```python
from build123d import *

# Parameters (mm, degrees)
SKETCH1_W                    = 60
SKETCH1_H                    = 170
BASE_FLANGE1_DEPTH           = 4
EDGE_FLANGE1_STRIP_W         = 26
EDGE_FLANGE1_STRIP_H         = 4
EDGE_FLANGE1_STRIP_CUT_DEPTH = 170
EDGE_FLANGE1_DEPTH           = 170
SKETCH15_R                   = 10
CUT_EXTRUDE4_DEPTH           = 10
CUT_EXTRUDE5_DEPTH           = 10
FILLET1_R                    = 10
F_1_0MM_DOWEL_HOLE2_D        = 5.2
F_1_0MM_DOWEL_HOLE2_DEPTH    = 12.03
F_1_0MM_DOWEL_HOLE2_TIP      = 1.562237609
SKETCH33_R                   = 2.6
CUT_EXTRUDE6_DEPTH           = 7
F_1_0MM_DOWEL_HOLE3_D        = 5.2
F_1_0MM_DOWEL_HOLE3_DEPTH    = 12.03
F_1_0MM_DOWEL_HOLE3_TIP      = 1.562237609
CUT_EXTRUDE7_DEPTH           = 10


# Sheet-metal steps are written as plain solids
with BuildPart() as part:
    # Sketch1 → Base-Flange1 (new body)
    with BuildSketch(Plane(origin=(0, 0, 0), x_dir=(1, 0, 0), z_dir=(0, 1, 0))):
        Rectangle(SKETCH1_W, SKETCH1_H)
    extrude(amount=-BASE_FLANGE1_DEPTH)

    # Edge-Flange1 strip (across the edge) → Edge-Flange1 strip cut (cut)
    with BuildSketch(Plane(origin=(-30, 0, -85), x_dir=(1, 0, 0), z_dir=(0, 0, 1))):
        with Locations((-8, -2)):
            Rectangle(EDGE_FLANGE1_STRIP_W, EDGE_FLANGE1_STRIP_H)
    extrude(amount=EDGE_FLANGE1_STRIP_CUT_DEPTH, mode=Mode.SUBTRACT)

    # Edge-Flange1 section (across the edge) → Edge-Flange1 (add)
    with BuildSketch(Plane(origin=(-30, 0, -85), x_dir=(1, 0, 0), z_dir=(0, 0, 1))):
        with BuildLine():
            Line((-4, 5), (-4, 186))
            Line((-4, 186), (0, 186))
            Line((0, 186), (0, 5))
            ThreePointArc((0, 5), (1.464466094, 1.464466094), (5, 0))
            Line((5, 0), (5, -4))
            ThreePointArc((5, -4), (-1.363961031, -1.363961031), (-4, 5))
        make_face()
    extrude(amount=EDGE_FLANGE1_DEPTH)

    # Sketch15 → Cut-Extrude4 (cut)
    with BuildSketch(Plane(origin=(-30, 0, 0), x_dir=(0, 0, -1), z_dir=(1, 0, 0))):
        with Locations(Location((-43, 63, 0), (0, 0, 90))):
            Circle(SKETCH15_R)
        with Locations(Location((57, 143, 0), (0, 0, 90))):
            Circle(SKETCH15_R)
    extrude(amount=-CUT_EXTRUDE4_DEPTH, mode=Mode.SUBTRACT)

    # Sketch16 → Cut-Extrude5 (cut)
    with BuildSketch(Plane(origin=(-30, 0, 0), x_dir=(0, 0, -1), z_dir=(1, 0, 0))):
        Polygon((-85, 96), (45, 186), (-85, 186), align=None)
    extrude(amount=-CUT_EXTRUDE5_DEPTH, mode=Mode.SUBTRACT)

    # Fillet1
    fillet1_edges = [part.edges().sort_by_distance(p)[0] for p in [
        (-32, 186, -85),
        (-32, 186, -45),
        (-32, 96, 85),
        (30, -2, 85),
        (30, -2, -85),
    ]]
    fillet(fillet1_edges, radius=FILLET1_R)

    # Ø1.0mm Dowel Hole2
    with Locations(Plane(origin=(-30, 0, 0), x_dir=(0, 0, -1), z_dir=(1, 0, 0))):
        with Locations((-72.5, 26), (72.5, 26), (72.5, 116), (-22.5, 101), (59.5, 178)):
            Hole(F_1_0MM_DOWEL_HOLE2_D / 2, depth=F_1_0MM_DOWEL_HOLE2_DEPTH)
            with Locations((0, 0, -(F_1_0MM_DOWEL_HOLE2_DEPTH + F_1_0MM_DOWEL_HOLE2_TIP / 2))):  # 118° drill point
                Cone(0, F_1_0MM_DOWEL_HOLE2_D / 2, F_1_0MM_DOWEL_HOLE2_TIP, mode=Mode.SUBTRACT)

    # Sketch33 → Cut-Extrude6 (cut)
    with BuildSketch(Plane(origin=(-30, 0, 0), x_dir=(0, 0, -1), z_dir=(1, 0, 0))):
        with Locations(Location((-10, 61.5, 0), (0, 0, 90))):
            Circle(SKETCH33_R)
        with Locations(Location((-76, 61.5, 0), (0, 0, 90))):
            Circle(SKETCH33_R)
        with Locations(Location((-43, 23, 0), (0, 0, 90))):
            Circle(SKETCH33_R)
    extrude(amount=-CUT_EXTRUDE6_DEPTH, mode=Mode.SUBTRACT)

    # Ø1.0mm Dowel Hole3
    with Locations(Plane(origin=(0, 0, 0), x_dir=(1, 0, 0), z_dir=(0, 1, 0))):
        with Locations((15, 70), (15, 0), (15, -70)):
            Hole(F_1_0MM_DOWEL_HOLE3_D / 2, depth=F_1_0MM_DOWEL_HOLE3_DEPTH)
            with Locations((0, 0, -(F_1_0MM_DOWEL_HOLE3_DEPTH + F_1_0MM_DOWEL_HOLE3_TIP / 2))):  # 118° drill point
                Cone(0, F_1_0MM_DOWEL_HOLE3_D / 2, F_1_0MM_DOWEL_HOLE3_TIP, mode=Mode.SUBTRACT)

    # Sketch36 → Cut-Extrude7 (cut)
    with BuildSketch(Plane(origin=(0, 0, 0), x_dir=(1, 0, 0), z_dir=(0, 1, 0))):
        with BuildLine():
            Line((11, 67.4), (19, 67.4))
            ThreePointArc((19, 67.4), (21.6, 70), (19, 72.6))
            Line((19, 72.6), (11, 72.6))
            ThreePointArc((11, 72.6), (8.4, 70), (11, 67.4))
        make_face()
        with BuildLine():
            Line((11, -2.6), (19, -2.6))
            ThreePointArc((19, -2.6), (21.6, 0), (19, 2.6))
            Line((19, 2.6), (11, 2.6))
            ThreePointArc((11, 2.6), (8.4, 0), (11, -2.6))
        make_face()
        with BuildLine():
            Line((11, -72.6), (19, -72.6))
            ThreePointArc((19, -72.6), (21.6, -70), (19, -67.4))
            Line((19, -67.4), (11, -67.4))
            ThreePointArc((11, -67.4), (8.4, -70), (11, -72.6))
        make_face()
    extrude(amount=-CUT_EXTRUDE7_DEPTH, mode=Mode.SUBTRACT)


solid = part.part
```
Model file for the job. Use its own axes, mm. A direction names the side the tool comes from. Round coordinates to 2 decimals unless told otherwise and drop trailing zeros. Order: outer loops, then holes, each group sorted by start corner. A loop starts at its lowest first (then second) coordinate and runs counter-clockwise, first axis right, second up. Notation, with made-up numbers: M 52,76 L 104,76 A19 cw 104,86 Z; hole C 80.5,-23.5 d3. An arc over 180 degrees is marked long. Use CSV: the item, a comma, the result in double quotes.
Item 1: Saw through at A-A (x = 15). List the corners of the cut face in (y, z), plus the area to 3 significant figures.
Worked answers:
outline,"M -4,-85 L 0,-85 L 0,-72.6 L -4,-72.6 Z; M -4,-67.4 L 0,-67.4 L 0,-2.6 L -4,-2.6 Z; M -4,2.6 L 0,2.6 L 0,67.4 L -4,67.4 Z; M -4,72.6 L 0,72.6 L 0,85 L -4,85 Z"
area,"618 mm²"
Item 2: Pull direction X, two halves, no side cores. Call faces 4 (the face through (21.6, -2, 70.1)), 5 (the face through (-31.972, 59.584, 77.757)), 6 (the face through (26.99, -2.03, -82.15)), 7 (the face through (15, -2, 72.6)): released by +X, released by -X, zero draft, split by the parting line, or undercut.
Worked answers:
face 4,"undercut"
face 5,"zero draft"
face 6,"released by +X"
face 7,"undercut"
Item 3: Saw through at B-B (y = 61.5). List the corners of the cut face in (x, z).
Worked answers:
outline,"M -34,-85 L -30,-85 L -30,7.4 L -34,7.4 Z; M -34,12.6 L -30,12.6 L -30,33.11 L -34,33.11 Z; M -34,52.89 L -30,52.89 L -30,73.4 L -34,73.4 Z; M -34,78.6 L -30,78.6 L -30,85 L -34,85 Z"
Item 4: Saw through at D-D (z = 0). List the corners of the cut face in (x, y), plus the area to 3 significant figures.
Worked answers:
outline,"M -34,5 A9 ccw -25,-4 L 8.4,-4 L 8.4,0 L -25,0 A5 cw -30,5 L -30,154.85 L -34,154.85 Z; M 21.6,-4 L 30,-4 L 30,0 L 21.6,0 Z"
area,"811 mm²"
Item 5: Pin check, flat tips, straight feed: pin 1 (7 mm diameter, centred on y = 116, z = -72.5, fed in from +X); pin 2 (12 mm diameter, centred on x = 1, z = 45.5, fed in from +Y). Stop position of each tip, or through.
Worked answers:
pin 1,"x = -30"
pin 2,"y = 0"
Item 6: Probe probe 1 along Y at (x, z) = (-30.9, -59.5); probe 2 along X at (y, z) = (92.5, 7.5); probe 3 along Y at (x, z) = (15, -25.5). List the from-to ranges inside material, lowest first.
Worked answers:
probe 1,"-1.8 to 133.32, 152.68 to 175.4, 180.6 to 186"
probe 2,"-34 to -30"
probe 3,"-4 to 0"
Item 7: Which spindle directions (+Z, -Z, +X, -X, +Y, -Y) get a long thin tool onto all of the face, cutting with end or side? Do faces 1 (the face through (8.4, -2, -70.1)), 2 (the face through (-32, 58.9, 10.1)), 3 (the face through (2, 0, -1)). Say none if no direction does.
Worked answers:
face 1,"+Y, -Y"
face 2,"+X, -X"
face 3,"+Z, -Z, +X, +Y"
Item 8: Saw through at C-C (y = 136). List the corners of the cut face in (x, z), plus the area to 3 significant figures.
Worked answers:
outline,"M -34,-85 L -30,-85 L -30,-64.14 L -34,-64.14 Z; M -34,-49.86 L -30,-49.86 L -30,27.22 L -34,27.22 Z"
area,"392 mm²"
